Check sheet for the modelled part. Datum: model origin and axes. Units: mm. A direction names the side the tool comes from. Round coordinates to 2 decimals unless told otherwise and drop trailing zeros. Write each loop counter-clockwise with the first axis right and the second up, starting at its lowest first coordinate (ties: lowest second). Pieces come first, ordered by that corner, then holes.
Item 1: Material ranges on line 1 (X direction, y = 22, z = 1.2); line 2 (Y direction, x = 4.5, z = 2.75); line 3 (X direction, y = 8, z = 1.95), recorded low to high.
Item 2: Tool access check on faces 4 (the flat face through (5.1, 1, 2)), 5 (the flat face through (8.1, 23, 2)), 6 (the cylindrical face through (7.799, 21.285, 2.535)). Record the directions out of +Z, -Z, +X, -X, +Y, -Y that give a thin tool (end or side, any length) a straight path to the whole face; none if there is none.
Item 3: Cross-section at B-B on z = 3.55. Enter the section's corners in (x, y).
Item 4: Release check for a two-part mould opening along Y. For faces 1 (the flat face through (-4, 12, 2)), 2 (the flat face through (2, -4, 2)), 3 (the cylindrical face through (5.385, 21.301, 2.535)) record: +Y half, -Y half, draft (parallel to the pull), parting line (faces both ways), or undercut.
Item 5: Cross-section at C-C on y = 15.5. Enter the section's corners in (x, z).
Item 6: Cross-section at D-D on x = 6.75. Enter the section's corners in (y, z), plus the area to 3 significant figures.
Item 7: Cross-section at A-A on x = 2.5. Enter the section's corners in (y, z), plus the area to 3 significant figures.
Item 8: Go/stop test with flat-tipped pins: pin 1 Ø1.1 at (x, z) = (6.5, 1.5) entering from -Y; pin 2 Ø1.5 at (y, z) = (14.5, 3.5) entering from +X. Record where each tip stops, or that it passes through.
from build123d import *

# Parameters (mm, degrees)
F1_DEPTH = 5
F2_R     = 3
F3_R     = 0.5
F4_R     = 1


with BuildPart() as f1:
    # F0 (on Top) → F1 (new body)
    with BuildSketch(Plane.XY):
        Polygon((5.1, 0), (0, 0), (0, 24), (5.1, 24), (5.1, 21), (8.1, 21), (8.1, 28), (-4, 28), (-4, -4), (8.1, -4), (8.1, 3), (5.1, 3), align=None)
    extrude(amount=F1_DEPTH)

    # F2
    f2_edges = [f1.edges().sort_by_distance(p)[0] for p in [
        (-4, 28, 2.5),
        (-4, -4, 2.5),
        (8.1, -4, 2.5),
        (8.1, 28, 2.5),
    ]]
    fillet(f2_edges, radius=F2_R)

    # F3
    f3_edges = [f1.edges().sort_by_distance(p)[0] for p in [
        (0, 24, 2.5),
        (5.1, 24, 2.5),
        (0, 0, 2.5),
        (5.1, 0, 2.5),
    ]]
    fillet(f3_edges, radius=F3_R)

    # F4
    f4_edges = [f1.edges().sort_by_distance(p)[0] for p in [
        (5.1, 21, 2.5),
        (5.1, 3, 2.5),
        (8.1, 21, 2.5),
        (8.1, 3, 2.5),
    ]]
    fillet(f4_edges, radius=F4_R)


solid = f1.part
Response values:
1. line 1: x = -4 to 0, 5.1 to 8.1
1. line 2: y = -4 to 0, 24 to 28
1. line 3: x = -4 to 0
2. face 4: +Z, -Z
2. face 5: +Z, -Z, +X, +Y, -Y
2. face 6: +Z, -Z, +X
3. outline: (-4, -1) arc R3 ccw to (-1, -4) - (5.1, -4) arc R3 ccw to (8.1, -1) - (8.1, 2) arc R1 ccw to (7.1, 3) - (6.1, 3) arc R1 ccw to (5.1, 2) - (5.1, 0.5) arc R0.5 cw to (4.6, 0) - (0.5, 0) arc R0.5 cw to (0, 0.5) - (0, 23.5) arc R0.5 cw to (0.5, 24) - (4.6, 24) arc R0.5 cw to (5.1, 23.5) - (5.1, 22) arc R1 ccw to (6.1, 21) - (7.1, 21) arc R1 ccw to (8.1, 22) - (8.1, 25) arc R3 ccw to (5.1, 28) - (-1, 28) arc R3 ccw to (-4, 25) - close
4. face 1: draft
4. face 2: -Y half
4. face 3: undercut
5. outline: (-4, 0) - (0, 0) - (0, 5) - (-4, 5) - close
6. outline: (-3.51, 0) - (3, 0) - (3, 5) - (-3.51, 5) - close; (21, 0) - (27.51, 0) - (27.51, 5) - (21, 5) - close
6. area: 65.1 mm2
7. outline: (-4, 0) - (0, 0) - (0, 5) - (-4, 5) - close; (24, 0) - (28, 0) - (28, 5) - (24, 5) - close
7. area: 40.0 mm2
8. pin 1: stops at y = -3.88
8. pin 2: stops at x = 0
